Here's how the part is built. I have some questions about the finished solid (model axes, mm). A direction names the side the tool comes from. Coordinates: 2 decimals unless noted, no trailing zeros. Loops run counter-clockwise (first coordinate to the right, second up) from the corner with the lowest first, then second, coordinate; pieces in that order, holes last.
```python
from build123d import *

# Parameters (mm, degrees)
SKETCH_R        = 17.5
SKETCH001_R     = 20
SKETCH002_R     = 4.75
POCKET_DEPTH    = 6.501
SKETCH003_R     = 2
POCKET001_DEPTH = 6.501
SKETCH004_R     = 3.5
POCKET002_DEPTH = 2.5
FILLET_R        = 0.5
SKETCH005_R     = 7.5
POCKET003_DEPTH = 4.5


with BuildPart() as part:
    # Sketch (on XY_Plane of Origin) → AdditiveLoft section 0
    with BuildSketch(Plane.XY):
        Circle(SKETCH_R)
    # Sketch001 (on Sketch) → AdditiveLoft section 1
    with BuildSketch(Plane.XY.offset(6.5)):
        Circle(SKETCH001_R)
    loft()

    # Sketch002 (on Face3 of AdditiveLoft) → Pocket (cut, through all)
    with BuildSketch(Plane.XY.offset(6.5)):
        Circle(SKETCH002_R)
    extrude(amount=-POCKET_DEPTH, mode=Mode.SUBTRACT)

    # Sketch003 (on Face1 of Pocket) → Pocket001 (cut, through all)
    with BuildSketch(Plane(origin=(0, 0, 0), x_dir=(1, 0, 0), z_dir=(0, 0, -1))):
        with Locations((-12.5, 0)):
            Circle(SKETCH003_R)
        with Locations((12.5, 0)):
            Circle(SKETCH003_R)
    extrude(amount=-POCKET001_DEPTH, mode=Mode.SUBTRACT)

    # Sketch004 (on Face6 of Pocket001) → Pocket002 (cut)
    with BuildSketch(Plane.XY.offset(6.5)):
        with Locations((-12.5, 0)):
            Circle(SKETCH004_R)
        with Locations((12.5, 0)):
            Circle(SKETCH004_R)
    extrude(amount=-POCKET002_DEPTH, mode=Mode.SUBTRACT)

    # Fillet
    fillet_edges = [part.edges().sort_by_distance(p)[0] for p in [
        (-20, 0, 6.5),
    ]]
    fillet(fillet_edges, radius=FILLET_R)

    # Sketch005 (on Face4 of Fillet) → Pocket003 (cut)
    with BuildSketch(Plane.XY.offset(6.5)):
        Circle(SKETCH005_R)
    extrude(amount=-POCKET003_DEPTH, mode=Mode.SUBTRACT)


solid = part.part
```
1. For pin 1 (9 mm diameter, centred on x = -12.5, y = 0, fed in from +Z); pin 2 (1 mm diameter, centred on x = 15.5, z = 2, fed in from +Y); pin 3 (3 mm diameter, centred on y = 12, z = 2.5, fed in from +X); pin 4 (1.5 mm diameter, centred on y = 14.5, z = 3, fed in from +X), each with a flat end and sliding along its axis, tell me the tip position at first contact or that it passes through.
2. I want a section at C-C (z = 1). Please give me the cut outline in (x, y), then the cut area to 3 significant figures.
3. I need wall thicknesses on line 1 along X through (y, z) = (-2, 4.5); line 2 along X through (y, z) = (3, 3.25); line 3 along X through (y, z) = (4, 4.25). Which ranges of each line are inside material? Lowest first, please.
4. We'd pull the mould along X, two halves only. Please class faces 3 (the flat face through (4, -4, 0)), 4 (the conical face through (-2.3, 17.49, 0.36)), 5 (the flat face through (14, -2, 4)), 6 (the flat face through (-11, -2, 4)): +X half, -X half, draft (parallel to the pull), parting line (faces both ways), or undercut.
5. I want a section at A-A (x = 0). Please give me the cut outline in (y, z).
6. On a 3-axis mill with a long thin cutter (end or side, diameter ignored), from which of +Z, -Z, +X, -X, +Y, -Y can I reach the whole of each face in a straight line? I mean faces 1 (the cylindrical face through (-7.493, 0.33, 4.281)), 2 (the cylindrical face through (10.9, 1.2, 2)). Say none if no direction works.
7. I want a section at B-B (y = 0). Give the number of separate pieces and of enclosed holes in the cut face, then the cut area to 3 significant figures.
Response values:
1. pin 1: stops at z = 6.5
1. pin 2: stops at y = 10.5
1. pin 3: stops at x = 15.4
1. pin 4: stops at x = 12.71
2. outline: circle Ø35.77 at (0, 0); hole circle Ø4 at (-12.5, 0); hole circle Ø9.5 at (0, 0); hole circle Ø4 at (12.5, 0)
2. area: 909 mm2
3. line 1: x = -19.13 to -15.37, -9.63 to -7.23, 7.23 to 9.63, 15.37 to 19.13
3. line 2: x = -18.51 to -6.87, 6.87 to 18.51
3. line 3: x = -18.71 to -6.34, 6.34 to 18.71
4. face 3: draft
4. face 4: parting line
4. face 5: undercut
4. face 6: undercut
5. outline: (-19.74, 5.82) - (-17.5, 0) - (-4.75, 0) - (-4.75, 2) - (-7.5, 2) - (-7.5, 6.5) - (-19.27, 6.5) arc R0.5 ccw to start; (4.75, 0) - (17.5, 0) - (19.74, 5.82) arc R0.5 ccw to (19.27, 6.5) - (7.5, 6.5) - (7.5, 2) - (4.75, 2) - close
6. face 1: +Z
6. face 2: +Z, -Z
7. separate pieces: 4
7. enclosed holes: 0
7. area: 90.0 mm2
